Autodesk Inventor part; units mm, degrees
ref_plane "YZ Plane" through (0, 0, 0) normal (1, 0, 0) x (0, 1, 0)
ref_plane "XZ Plane" through (0, 0, 0) normal (0, 1, 0) x (-1, 0, 0)
ref_plane "XY Plane" through (0, 0, 0) normal (0, 0, 1) x (1, 0, 0)
sketch "Sketch1" plane through (0, 0, 0) normal (0, 0, 1) x (1, 0, 0)
  circle A0 centre (0, 0) radius 2.159
  circle A1 centre (0, 0) radius 12.7
  line L0 (0, 0) -> (0, 38.1) construction
  line L1 (0, 38.1) -> (12.827, 38.1) construction
  line L2 (12.827, 38.1) -> (12.827, 53.975)
  line L3 (12.827, 53.975) -> (30.7875, 71.9355)
  line L4 (12.827, 53.975) -> (38.227, 53.975) construction
  arc A2 (38.227, 53.975) -> (30.7875, 71.9355) centre (12.827, 53.975) ccw
  line L5 (12.827, 38.1) -> (-10.1397, 7.647)
  arc A3 (33.1064, 22.806) -> (38.227, 38.1) centre (12.827, 38.1) ccw
  line L6 (33.1064, 22.806) -> (10.1397, -7.647)
  line L7 (38.227, 38.1) -> (38.227, 53.975)
  circle A4 centre (31.877, 53.975) radius 2.159
  circle A5 centre (19.177, 53.975) radius 2.159
  circle A6 centre (31.877, 41.275) radius 2.159
  circle A7 centre (19.177, 41.275) radius 2.159
  circle A8 centre (31.877, 53.975) radius 6.35 construction
  circle A9 centre (19.177, 53.975) radius 6.35 construction
  circle A10 centre (19.177, 28.575) radius 2.159
  circle A11 centre (19.177, 15.875) radius 2.159
  dimension "d0" = 4.318
  dimension "d1" = 25.4
  dimension "d2" = 38.1
  dimension "d3" = 12.827
  dimension "d4" = 15.875
  dimension "d5" = 25.4
  dimension "d6" = 45
  dimension "d7" = 4.318
  dimension "d10" = 12.7
  dimension "d13" = 12.7
  dimension "d17" = 12.7
  dimension "d18" = 12.7
extrude "Extrusion1" add sketch "Sketch1" along normal blind 3
fillet "Fillet1" radius 6.35 3 edges at (30.7875, 71.9355, 1.5) (12.827, 53.975, 1.5) (12.827, 38.1, 1.5)
properties part number "IntakeAftArm"
Part model, mm, in its own coordinate system. Give positions to 0.01 mm unless a question says otherwise; leave off trailing zeros. Order: outer loops, then holes, each group sorted by start corner. A loop starts at its lowest first (then second) coordinate and runs counter-clockwise, first axis right, second up. Notation, with made-up numbers: M -27,21.25 L 18,21.25 A24 ccw 18,36.25 Z; hole C -24.75,28 d10. An arc over 180 degrees is marked long. Use a Markdown table: item, result. Add a question column.
(1) Saw through at C-C, the plane z = 1.15. Give the number of separate pieces and of enclosed holes in the cut face, and give its area (3 significant figures).
(2) Saw through at B-B, the plane y = 0. Give the cut face in (x, z).
(3) Probe line 1 along X through (y, z) = (39.5, 2.4); line 2 along X through (y, z) = (43, 2.2); line 3 along Y through (x, z) = (20, 2.45). List the from-to ranges inside material, lowest first. Write a range as [from, to].
(4) Mould opens along X. For faces 1 (the face through (18.709, 43.383, 1.479)), 2 (the face through (12.827, 46, 1)), 3 (the face through (36.949, 30.145, 1.479)) say: +X half, -X half, draft (parallel to the pull), parting line (faces both ways), or undercut.
(5) Saw through at D-D, the plane x = -9. Give the cut face in (y, z), and give its area (3 significant figures).
(6) Saw through at A-A, the plane x = 0. Give the cut face in (y, z).
(7) Drop flat-ended pins along their axis: P1, Ø7, axis at x = 19.177, y = 41.275, coming from the -Z side; P2, Ø6, axis at x = -6.5, y = 21, coming from the +Z side; P3, Ø0.9, axis at y = 44.5, z = 1.5, coming from the -X side. Give the stop position or say it passes through.
Answer key:
| question | item | result |
|---|---|---|
| 1 | separate pieces | 1 |
| 1 | enclosed holes | 7 |
| 1 | area | 1,970 mm^2 |
| 2 | outline | M -12.7,0 L -2.16,0 L -2.16,3 L -12.7,3 Z; M 2.16,0 L 15.91,0 L 15.91,3 L 2.16,3 Z |
| 3 | line 1 | [12.79, 17.95], [20.41, 30.65], [33.11, 38.23] |
| 3 | line 2 | [12.83, 17.88], [20.48, 30.58], [33.18, 38.23] |
| 3 | line 3 | [5.43, 13.88], [17.87, 26.58], [30.57, 39.28], [43.27, 51.98], [55.97, 61.15] |
| 4 | face 1 | undercut |
| 4 | face 2 | -X half |
| 4 | face 3 | +X half |
| 5 | outline | M -8.96,0 L 9.16,0 L 9.16,3 L -8.96,3 Z |
| 5 | area | 54.4 mm^2 |
| 6 | outline | M -12.7,0 L -2.16,0 L -2.16,3 L -12.7,3 Z; M 2.16,0 L 21.09,0 L 21.09,3 L 2.16,3 Z |
| 7 | P1 | z = 0 |
| 7 | P2 | through |
| 7 | P3 | x = 12.83 |
